Autodesk Fusion 360 part; units mm, degrees
sketch "Sketch1" plane through (0, 0, 0) normal (0, 0, 1) x (1, 0, 0)
  line L0 (3.81, 0) -> (113.03, 0)
  line L1 (116.84, 3.81) -> (116.84, 68.58)
  line L2 (113.03, 72.39) -> (3.81, 72.39)
  line L3 (0, 68.58) -> (0, 3.81)
  arc A0 (0, 3.81) -> (3.81, 0) centre (3.81, 3.81) ccw
  arc A1 (113.03, 0) -> (116.84, 3.81) centre (113.03, 3.81) ccw
  arc A2 (116.84, 68.58) -> (113.03, 72.39) centre (113.03, 68.58) ccw
  arc A3 (3.81, 72.39) -> (0, 68.58) centre (3.81, 68.58) ccw
  circle A4 centre (15.24, 12.7) radius 1.905
  circle A5 centre (101.6, 12.7) radius 1.905
  circle A6 centre (101.6, 59.69) radius 1.905
  circle A7 centre (15.24, 59.69) radius 1.905
  point P0 (116.84, 0)
  point P1 (0, 72.39)
  dimension "d1" = 116.84
  dimension "d2" = 72.39
  dimension "d3" = 3.81
  dimension "d4" = 3.81
  dimension "d5" = 3.81
  dimension "d6" = 3.81
  dimension "d7" = 3.81
  dimension "d8" = 15.24
  dimension "d9" = 12.7
  dimension "d10" = 3.81
  dimension "d11" = 3.81
  dimension "d12" = 3.81
extrude "Extrude1" add sketch "Sketch1" along normal blind 3.048
sketch "Sketch2" plane through (0, 0, 0) normal (0, 0, -1) x (1, 0, 0)
  circle A0 centre (15.24, -59.69) radius 1.905
  circle A1 centre (101.6, -59.69) radius 1.905
  circle A2 centre (15.24, -12.7) radius 1.905
  circle A3 centre (101.6, -12.7) radius 1.905
  arc A4 (0, -68.58) -> (3.81, -72.39) centre (3.81, -68.58) ccw
  line L0 (3.81, -72.39) -> (113.03, -72.39)
  arc A5 (113.03, -72.39) -> (116.84, -68.58) centre (113.03, -68.58) ccw
  line L1 (116.84, -68.58) -> (116.84, -3.81)
  arc A6 (116.84, -3.81) -> (113.03, 0) centre (113.03, -3.81) ccw
  line L2 (113.03, 0) -> (3.81, 0)
  arc A7 (3.81, 0) -> (0, -3.81) centre (3.81, -3.81) ccw
  line L3 (0, -3.81) -> (0, -68.58)
  line L4 (34.29, -22.695) -> (64.77, -22.695)
  line L5 (64.77, -22.695) -> (64.77, -49.695)
  line L6 (64.77, -49.695) -> (34.29, -49.695)
  line L7 (34.29, -49.695) -> (34.29, -22.695)
  circle A8 centre (88.9518, -36.0108) radius 3.175
  line L8 (0, -36.195) -> (116.84, -36.195) construction
  line L9 (35.306, -26.695) -> (54.306, -26.695)
  line L10 (54.306, -26.695) -> (54.306, -45.695)
  line L11 (54.306, -45.695) -> (35.306, -45.695)
  line L12 (35.306, -45.695) -> (35.306, -26.695)
  line L13 (35.306, -26.695) -> (54.306, -45.695) construction
  line L14 (54.306, -26.695) -> (35.306, -45.695) construction
  circle A9 centre (35.814, -24.765) radius 1.016
  circle A10 centre (38.354, -24.765) radius 1.016
  circle A11 centre (40.894, -24.765) radius 1.016
  circle A12 centre (43.434, -24.765) radius 1.016
  circle A13 centre (45.974, -24.765) radius 1.016
  circle A14 centre (48.514, -24.765) radius 1.016
  circle A15 centre (51.054, -24.765) radius 1.016
  circle A16 centre (53.594, -24.765) radius 1.016
  circle A17 centre (35.814, -47.625) radius 1.016
  circle A18 centre (38.354, -47.625) radius 1.016
  circle A19 centre (40.894, -47.625) radius 1.016
  circle A20 centre (43.434, -47.625) radius 1.016
  circle A21 centre (45.974, -47.625) radius 1.016
  circle A22 centre (48.514, -47.625) radius 1.016
  circle A23 centre (51.054, -47.625) radius 1.016
  circle A24 centre (53.594, -47.625) radius 1.016
  point P0 (44.806, -36.195)
  dimension "d15" = 30.48
  dimension "d16" = 27
  dimension "d18" = 34.29
  dimension "d19" = 6.35
  dimension "d20" = 19
  dimension "d21" = 19
  dimension "d22" = 1.016
  dimension "d23" = 2.032
  dimension "d26" = 2.54
  dimension "d27" = -22.86
  dimension "d29" = 1.524
  dimension "d37" = 11.43
extrude "Extrude2" cut sketch "Sketch2" against normal through all contours L9 L10 L11 L12
extrude "Extrude3" cut sketch "Sketch2" against normal blind 2.032 contours A9 | A10 | A11 | A12 | A13 | A14 | A15 | A16 | A17 | A18 | A19 | A20 | A21 | A22 | A23 | A24
extrude "Extrude4" cut sketch "Sketch2" against normal blind 1.016 contours L4 L5 L6 L7
extrude "Extrude5" cut sketch "Sketch2" against normal through all contours A8
Verification items for the finished model (mm, model axes). Give positions to 0.01 mm unless a question says otherwise; leave off trailing zeros. Write each loop counter-clockwise with the first axis right and the second up, starting at its lowest first coordinate (ties: lowest second). Pieces come first, ordered by that corner, then holes. Notation, with made-up numbers: (50.25, 46) -> (82.25, 46) arc R24 ccw to (82.25, 82) -> close; hole circle Ø10 at (87, 14.25). An arc over 180 degrees is marked (long way). Use CSV: the item, a comma, the result in double quotes.
(1) Sectioned sample at B-B (y = 59.69). Record the cut outline in (x, z) (3 decimals).
Derived:
outline,"(0, 0) -> (13.335, 0) -> (13.335, 3.048) -> (0, 3.048) -> close; (17.145, 0) -> (99.695, 0) -> (99.695, 3.048) -> (17.145, 3.048) -> close; (103.505, 0) -> (116.84, 0) -> (116.84, 3.048) -> (103.505, 3.048) -> close"
(2) Release check for a two-part mould opening along Y. For faces 1 (the flat face through (58, 37, 3.048)), 2 (the flat face through (56, 33, 1.016)), 3 (the flat face through (59, 72.39, 2)) record: +Y half, -Y half, draft (parallel to the pull), parting line (faces both ways), or undercut.
Derived:
face 1,"draft"
face 2,"undercut"
face 3,"+Y half"
(3) Sectioned sample at A-A (x = 101.6). Record the cut outline in (y, z) (3 decimals), plus the area to 3 significant figures.
Derived:
outline,"(0, 0) -> (10.795, 0) -> (10.795, 3.048) -> (0, 3.048) -> close; (14.605, 0) -> (57.785, 0) -> (57.785, 3.048) -> (14.605, 3.048) -> close; (61.595, 0) -> (72.39, 0) -> (72.39, 3.048) -> (61.595, 3.048) -> close"
area,"197 mm^2"
(4) Sectioned sample at C-C (z = 2.55). Record the cut outline in (x, y) (3 decimals), plus the area to 3 significant figures.
Derived:
outline,"(0, 3.81) arc R3.81 ccw to (3.81, 0) -> (113.03, 0) arc R3.81 ccw to (116.84, 3.81) -> (116.84, 68.58) arc R3.81 ccw to (113.03, 72.39) -> (3.81, 72.39) arc R3.81 ccw to (0, 68.58) -> close; hole circle Ø3.81 at (15.24, 12.7); hole circle Ø3.81 at (15.24, 59.69); hole (35.306, 26.695) -> (54.306, 26.695) -> (54.306, 45.695) -> (35.306, 45.695) -> close; hole circle Ø6.35 at (88.952, 36.011); hole circle Ø3.81 at (101.6, 12.7); hole circle Ø3.81 at (101.6, 59.69)"
area,"8,010 mm^2"
(5) Material ranges on L1, parallel to Y at x = 15.24, z = 2.35 (3 decimals); L2, parallel to X at y = 60, z = 2.6; L3, parallel to Y at x = 100.5, z = 2.35, recorded low to high.
Derived:
L1,"y = 0 to 10.795, 14.605 to 57.785, 61.595 to 72.39"
L2,"x = 0 to 13.36, 17.12 to 99.72, 103.48 to 116.84"
L3,"y = 0 to 11.14, 14.26 to 58.13, 61.25 to 72.39"
(6) Go/stop test with flat-tipped pins: pin 1 (1.6 mm diameter, centred on x = 35.814, y = 47.625, fed in from -Z); pin 2 (1.6 mm diameter, centred on x = 35.5, y = 25, fed in from -Z); pin 3 (3 mm diameter, centred on x = 101.6, y = 12.7, fed in from +Z). Record where each tip stops, or that it passes through.
Derived:
pin 1,"stops at z = 2.03"
pin 2,"stops at z = 1.02"
pin 3,"passes through"
